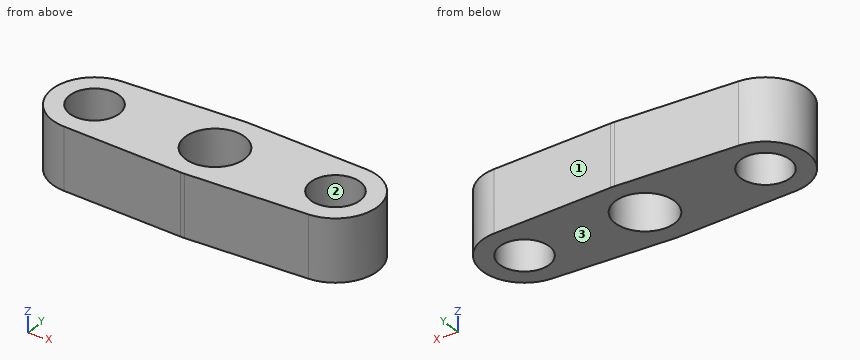
```python
from build123d import *

# Parameters (mm, degrees)
PAD_DEPTH     = 25
SKETCH001_R   = 12
SKETCH001_R_2 = 10
POCKET_DEPTH  = 25


with BuildPart() as part:
    # Sketch → Pad (new body)
    with BuildSketch(Plane.XY):
        with BuildLine():
            ThreePointArc((-48.708302, 16.985238), (-65, 1.6e-05), (-48.708334, -16.985237))
            Line((-48.708334, -16.985237), (-0.791666, -18.9835))
            ThreePointArc((-0.791666, -18.9835), (0, -19), (0.791666, -18.9835))
            Line((0.791666, -18.9835), (48.708335, -16.985237))
            ThreePointArc((48.708335, -16.985237), (65, 1e-06), (48.708333, 16.985237))
            Line((0.791666, 18.9835), (48.708333, 16.985237))
            ThreePointArc((0.791666, 18.9835), (0, 19), (-0.791667, 18.9835))
            Line((-48.708302, 16.985238), (-0.791667, 18.9835))
        make_face()
    extrude(amount=PAD_DEPTH)

    # Sketch001 (on Face10 of Pad) → Pocket (cut)
    with BuildSketch(Plane.XY.offset(25)):
        Circle(SKETCH001_R)
        with Locations((48, 0)):
            Circle(SKETCH001_R_2)
        with Locations((-48, 0)):
            Circle(SKETCH001_R_2)
    extrude(amount=-POCKET_DEPTH, mode=Mode.SUBTRACT)


solid = part.part
```
Could you check a few things on this model? Use its own coordinates, in mm. Face numbers are marked on the shaded views. Coordinates: 2 decimals unless noted, no trailing zeros. Write each loop counter-clockwise with the first axis right and the second up, starting at its lowest first coordinate (ties: lowest second). Pieces come first, ordered by that corner, then holes. Notation, with made-up numbers: (1, 12) -> (57, 12) arc R25 ccw to (57, 33) -> close; hole circle Ø2 at (45, 5.25). An arc over 180 degrees is marked (long way). Return JSON: item names as keys, results as strings.
(1) Imagine slicing it at B-B, the plane y = 0. Please give me the cut outline in (x, z).
Numbers:
{"outline": "(-65, 0) -> (-58, 0) -> (-58, 25) -> (-65, 25) -> close; (-38, 0) -> (-12, 0) -> (-12, 25) -> (-38, 25) -> close; (12, 0) -> (38, 0) -> (38, 25) -> (12, 25) -> close; (58, 0) -> (65, 0) -> (65, 25) -> (58, 25) -> close"}
(2) I need wall thicknesses on L1, parallel to X at y = -1.5, z = 18.5; L2, parallel to Y at x = 48, z = 17.5; L3, parallel to X at y = 4.5, z = 13.75. Which ranges of each line are inside material? Lowest first, please.
Numbers:
{"L1": "x = -64.93 to -57.89, -38.11 to -11.91, 11.91 to 38.11, 57.89 to 64.93", "L2": "y = -17.01 to -10, 10 to 17.01", "L3": "x = -64.39 to -56.93, -39.07 to -11.12, 11.12 to 39.07, 56.93 to 64.39"}
(3) Imagine slicing it at C-C, the plane x = -51. Please give me the cut outline in (y, z), then the cut area to 3 significant figures.
Numbers:
{"outline": "(-16.73, 0) -> (-9.54, 0) -> (-9.54, 25) -> (-16.73, 25) -> close; (9.54, 0) -> (16.73, 0) -> (16.73, 25) -> (9.54, 25) -> close", "area": "360 mm2"}
(4) Imagine slicing it at A-A, the plane z = 21. Please give me the cut outline in (x, y).
Numbers:
{"outline": "(-48.71, -16.99) -> (-0.79, -18.98) arc R19 ccw to (0.79, -18.98) -> (48.71, -16.99) arc R17 ccw to (48.71, 16.99) -> (0.79, 18.98) arc R19 ccw to (-0.79, 18.98) -> (-48.71, 16.99) arc R17 ccw to start; hole circle Ø20 at (-48, 0); hole circle Ø24 at (0, 0); hole circle Ø20 at (48, 0)"}
(5) Imagine slicing it at D-D, the plane y = 8.5. Please give me the cut outline in (x, z).
Numbers:
{"outline": "(-62.72, 0) -> (-53.27, 0) -> (-53.27, 25) -> (-62.72, 25) -> close; (-42.73, 0) -> (-8.47, 0) -> (-8.47, 25) -> (-42.73, 25) -> close; (8.47, 0) -> (42.73, 0) -> (42.73, 25) -> (8.47, 25) -> close; (53.27, 0) -> (62.72, 0) -> (62.72, 25) -> (53.27, 25) -> close"}
(6) I'm going to push flat-ended pins straight in: pin 1 (5 mm diameter, centred on x = -18, z = 16, fed in from -Y); pin 2 (1 mm diameter, centred on x = -42, z = 6, fed in from +Y); pin 3 (3 mm diameter, centred on y = -11, z = 9.5, fed in from -X). Where does each tip first touch, or does it pass through?
Numbers:
{"pin 1": "stops at y = -18.37", "pin 2": "stops at y = 17.29", "pin 3": "stops at x = -62.1"}
(7) We'd pull the mould along X, two halves only. Please class the marked faces 1, 2 and 3: +X half, -X half, draft (parallel to the pull), parting line (faces both ways), or undercut.
Numbers:
{"face 1": "+X half", "face 2": "undercut", "face 3": "draft"}
